Geometry: final body of the model. Coordinates: model frame, mm. Face numbers are marked on the shaded views. A direction names the side the tool comes from. Give positions to 0.01 mm unless a question says otherwise; leave off trailing zeros. Write each loop counter-clockwise with the first axis right and the second up, starting at its lowest first coordinate (ties: lowest second). Pieces come first, ordered by that corner, then holes.
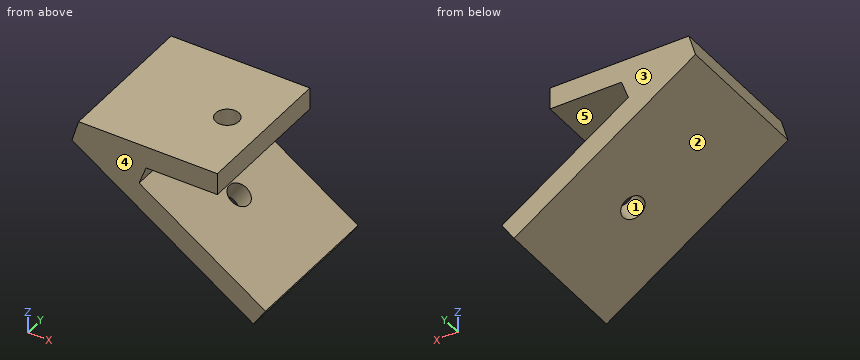
```python
from build123d import *

# Parameters (mm, degrees)
EXTRUDE_1_DEPTH     = 20
SKETCH_4_R          = 1.6
CUT_EXTRUDE_1_DEPTH = 4
CUT_EXTRUDE_2_REACH = 19.261
SKETCH_5_R          = 1.6


with BuildPart() as part:
    # 草图1 → 凸台-拉伸1 (new body)
    with BuildSketch(Plane(origin=(0, 0, 0), x_dir=(1, 0, 0), z_dir=(0, 1, 0))):
        Polygon((3.90131241, 80.330794947), (22.992985496, 80.330794947), (22.992985496, 83.330794947), (13.176134515, 83.330794947), (12.229840324, 85.890335427), (29.611004769, 97.487035171), (27.954494327, 99.971800834), (2.992985496, 83.330794947), align=None)
    extrude(amount=EXTRUDE_1_DEPTH)

    # 草图4 → 切除-拉伸1 (cut, through all)
    with BuildSketch(Plane(origin=(0, 0, -83.330794947), x_dir=(-1, 0, 0), z_dir=(0, 0, -1))):
        with Locations((-17.992985496, 10)):
            Circle(SKETCH_4_R)
    extrude(amount=-CUT_EXTRUDE_1_DEPTH, mode=Mode.SUBTRACT)

    # 草图5 → 切除-拉伸2 (cut, up to next)
    with BuildSketch(Plane(origin=(-37.539448284, 0, -56.309172427), x_dir=(-0.832050294, 0, 0.554700196), z_dir=(-0.554700196, 0, -0.832050294)), mode=Mode.PRIVATE) as cut_extrude_2_sk1:
        with Locations((-66.713922772, 10)):
            Circle(SKETCH_5_R)
    cut_extrude_2_tool1 = extrude(cut_extrude_2_sk1.sketch, amount=-CUT_EXTRUDE_2_REACH, mode=Mode.PRIVATE) & part.part
    add(cut_extrude_2_tool1.solids().sort_by_distance((17.969891, 10, -93.315398))[0], mode=Mode.SUBTRACT)


solid = part.part
```
Item 1: Line query: L1, parallel to Z at x = 18.25, y = 14; L2, parallel to Z at x = 25.5, y = 9.25; L3, parallel to X at y = 12.75, z = -90.5. Output: solid intervals per line, ascending.
Found:
L1: z = -93.5 to -89.91, -83.33 to -80.33
L2: z = -98.34 to -94.74
L3: x = 13.75 to 19.14
Item 2: Section D-D, the plane z = -82.75. Return the cut outline in (x, y), plus the area to 3 significant figures.
Found:
outline: (3.17, 0) - (22.99, 0) - (22.99, 20) - (3.17, 20) - close; hole circle Ø3.2 at (17.99, 10)
area: 388 mm2
Item 3: Section B-B, the plane y = 13. Return the cut outline in (x, z).
Found:
outline: (2.99, -83.33) - (27.95, -99.97) - (29.61, -97.49) - (12.23, -85.89) - (13.18, -83.33) - (22.99, -83.33) - (22.99, -80.33) - (3.9, -80.33) - close
Item 4: Pin query (flat end, axial travel): pin 1 Ø1 at (y, z) = (3.5, -83) entering from +X; pin 2 Ø3 at (x, y) = (15.5, 4) entering from -Z; pin 3 Ø6 at (y, z) = (14, -86.5) entering from -X. Return the tip coordinate at first contact, or that it passes through.
Found:
pin 1: stops at x = 22.99
pin 2: stops at z = -92.67
pin 3: stops at x = 3.25
Item 5: Pull-direction query (Y, two-part tool) for the marked faces 1, 2 and 3; classes: +Y half, -Y half, draft (parallel to the pull), parting line (faces both ways), or undercut.
Found:
face 1: undercut
face 2: draft
face 3: +Y half
Item 6: Section A-A, the plane y = 10. Return the cut outline in (x, z).
Found:
outline: (2.99, -83.33) - (16.64, -92.43) - (18.3, -89.94) - (12.23, -85.89) - (13.18, -83.33) - (16.39, -83.33) - (16.39, -80.33) - (3.9, -80.33) - close; (19.3, -94.2) - (27.95, -99.97) - (29.61, -97.49) - (20.96, -91.71) - close; (19.59, -83.33) - (22.99, -83.33) - (22.99, -80.33) - (19.59, -80.33) - close
Item 7: Reachability of the marked faces 4 and 5 from +Z, -Z, +X, -X, +Y, -Y: full face, straight path, thin tool, end or side. Return the list, or none.
Found:
face 4: +Z, -Z, +X, -X, -Y
face 5: +X, +Y, -Y
Item 8: Section C-C, the plane x = 13.5. Return the cut outline in (y, z), plus the area to 3 significant figures.
Found:
outline: (0, -90.34) - (20, -90.34) - (20, -86.74) - (0, -86.74) - close; (0, -83.33) - (20, -83.33) - (20, -80.33) - (0, -80.33) - close
area: 132 mm2
